Could you check a few things on this model? Use its own coordinates, in mm. Coordinates: 2 decimals unless noted, no trailing zeros. Order: outer loops, then holes, each group sorted by start corner. A loop starts at its lowest first (then second) coordinate and runs counter-clockwise, first axis right, second up. Notation, with made-up numbers: M 3.25,25.25 L 54.25,25.25 A13 ccw 54.25,29.25 Z; hole C 61,63 d5. An arc over 180 degrees is marked long. Put each result on its own line as item: value. Start each with the question number.
```python
from build123d import *

# Parameters (mm, degrees)
SKETCH_1_R      = 2
EXTRUDE_2_DEPTH = 40


with BuildPart() as part:
    # 草图1 → 凸台-拉伸2 (new body)
    with BuildSketch(Plane(origin=(0, 0, 0), x_dir=(1, 0, 0), z_dir=(0, 1, 0))):
        Polygon((-1.73, 3), (1.73, 3), (1.732050808, 3), (1.733076211, 2.998223949), (3.463076211, 0.001776051), (3.464101615, 0), (3.463076211, -0.001776051), (1.733076211, -2.998223949), (1.732050808, -3), (1.73, -3), (-1.73, -3), (-1.732050808, -3), (-1.733076211, -2.998223949), (-3.463076211, -0.001776051), (-3.464101615, 0), (-3.463076211, 0.001776051), (-1.733076211, 2.998223949), (-1.732050808, 3), align=None)
        with Locations(Location((0, 0, 0), (0, 0, 270))):
            Circle(SKETCH_1_R, mode=Mode.SUBTRACT)
    extrude(amount=EXTRUDE_2_DEPTH)


solid = part.part
```
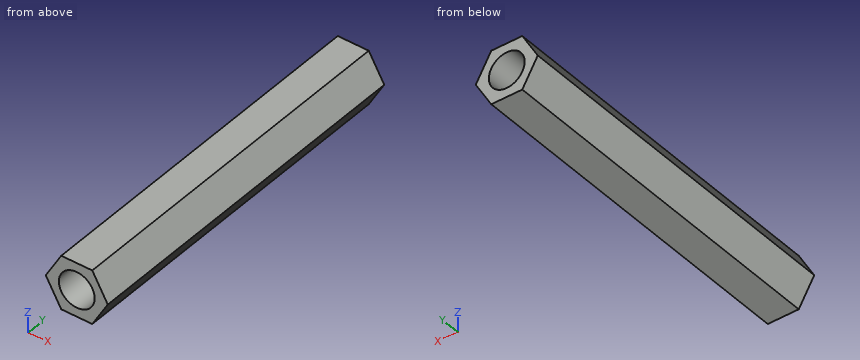
Item 1: I need wall thicknesses on probe 1 along Z at (x, y) = (-1, 11.5); probe 2 along X at (y, z) = (32, -1.4); probe 3 along Z at (x, y) = (-0.25, 7). Which ranges of each line are inside material? Lowest first, please.
Item 2: If we section it at A-A on x = 0: Write out the boundary of the cut face in (y, z), then the cut area to 3 significant figures.
Item 3: If we section it at D-D on x = 2.75: Write out the boundary of the cut face in (y, z).
Item 4: If we section it at C-C on z = -0.55: Write out the boundary of the cut face in (x, y).
Item 5: For pin 1 Ø2 at (x, z) = (1, 1.5) entering from +Y; pin 2 Ø2 at (y, z) = (18.5, -1.5) entering from +X, each with a flat end and sliding along its axis, tell me the tip position at first contact or that it passes through.
Geometry check:
1. probe 1: z = -3 to -1.73, 1.73 to 3
1. probe 2: x = -2.66 to -1.43, 1.43 to 2.66
1. probe 3: z = -3 to -1.98, 1.98 to 3
2. outline: M 0,-3 L 40,-3 L 40,-2 L 0,-2 Z; M 0,2 L 40,2 L 40,3 L 0,3 Z
2. area: 80.0 mm²
3. outline: M 0,-1.24 L 40,-1.24 L 40,1.24 L 0,1.24 Z
4. outline: M -3.15,0 L -1.92,0 L -1.92,40 L -3.15,40 Z; M 1.92,0 L 3.15,0 L 3.15,40 L 1.92,40 Z
5. pin 1: stops at y = 40
5. pin 2: stops at x = 3.18
